Geometry: final body of the model. Coordinates: model frame, mm. Round coordinates to 2 decimals unless told otherwise and drop trailing zeros. Loops run counter-clockwise (first coordinate to the right, second up) from the corner with the lowest first, then second, coordinate; pieces in that order, holes last. Notation, with made-up numbers: M -2.5,-33.75 L 41.5,-33.75 A20 cw 41.5,-24.75 Z; hole C -9.5,-22 d3. An arc over 180 degrees is marked long. Write each question's results on one line, items separated by ' | '.
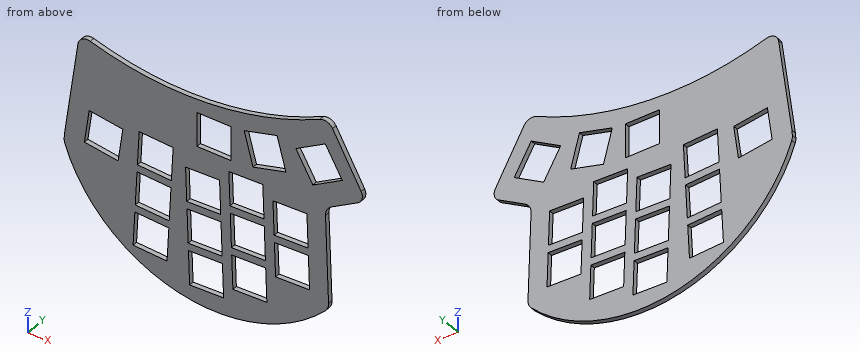
```python
from build123d import *

# Parameters (mm, degrees)
SKETCH1_W           = 14
SKETCH1_H           = 14
BOSS_EXTRUDE1_DEPTH = 2
FILLET1_R           = 5


with BuildPart() as part:
    # Sketch1 → Boss-Extrude1 (new body)
    with BuildSketch(Plane(origin=(0, 0, 0), x_dir=(1, 0, 0), z_dir=(0, 1, 0))):
        with BuildLine():
            Line((-10.586983819, 42.383324584), (-5.046266953, 2.959075179))
            ThreePointArc((-5.046266953, 2.959075179), (-3.174441029, 0.368828473), (0, 0))
            ThreePointArc((0, 0), (47.971062986, 5.333423777), (94.542026123, -7.347809821))
            ThreePointArc((94.542026123, -7.347809821), (97.488396157, -7.568143239), (99.777690602, -5.700317192))
            Line((99.777690602, -5.700317192), (111.550095971, 15.354261283))
            ThreePointArc((111.550095971, 15.354261283), (112.008410414, 17.939225635), (110.765402582, 20.251589006))
            Line((110.765402582, 20.251589006), (96.765402582, 28.334492774))
            Line((96.765402582, 28.334492774), (98.196951267, 69.32867968))
            ThreePointArc((98.196951267, 69.32867968), (36.880667069, 88.690951376), (-10.814532638, 45.566107052))
            Line((-10.814532638, 45.566107052), (-10.586983819, 42.383324584))
        make_face()
        Polygon((-0.449562029, 28.794432983), (13.414190971, 30.742856383), (11.465767571, 44.606609383), (-2.397985429, 42.658185983), align=None, mode=Mode.SUBTRACT)
        Polygon((20.152865671, 28.899486483), (34.133679071, 29.632189883), (33.400975671, 43.613003283), (19.420162271, 42.880299883), align=None, mode=Mode.SUBTRACT)
        Polygon((19.263154371, 45.876188583), (33.243967771, 46.608891983), (32.511264371, 60.589705383), (18.530450971, 59.857001983), align=None, mode=Mode.SUBTRACT)
        Polygon((18.373443071, 62.852890683), (32.354256471, 63.585594083), (31.621553071, 77.566407483), (17.640739671, 76.833704083), align=None, mode=Mode.SUBTRACT)
        Polygon((39.247799271, 35.544672383), (53.239270871, 35.056079383), (53.727863871, 49.047550983), (39.736392271, 49.536143983), align=None, mode=Mode.SUBTRACT)
        Polygon((39.841090671, 52.534316483), (53.832562271, 52.045723483), (54.321155271, 66.037195083), (40.329683671, 66.525788083), align=None, mode=Mode.SUBTRACT)
        Polygon((40.434382071, 69.523960583), (54.425853671, 69.035367583), (54.914446671, 83.026839183), (40.922975071, 83.515432183), align=None, mode=Mode.SUBTRACT)
        Polygon((57.062336771, 29.919527383), (71.053808371, 29.430934383), (71.542401371, 43.422405983), (57.550929771, 43.910998983), align=None, mode=Mode.SUBTRACT)
        Polygon((57.655628171, 46.909171483), (71.647099771, 46.420578483), (72.135692771, 60.412050083), (58.144221171, 60.900643083), align=None, mode=Mode.SUBTRACT)
        Polygon((58.248919571, 63.898815583), (72.240391171, 63.410222583), (72.728984171, 77.401694183), (58.737512571, 77.890287183), align=None, mode=Mode.SUBTRACT)
        Polygon((75.229359071, 34.388229583), (89.220830671, 33.899636583), (89.709423671, 47.891108183), (75.717952071, 48.379701183), align=None, mode=Mode.SUBTRACT)
        Polygon((75.822650471, 51.377873683), (89.814122071, 50.889280683), (90.302715071, 64.880752283), (76.311243471, 65.369345283), align=None, mode=Mode.SUBTRACT)
        with Locations((50.981291271, 18.033609783)):
            Rectangle(SKETCH1_W, SKETCH1_H, mode=Mode.SUBTRACT)
        Polygon((63.408077171, 10.383862283), (76.931038771, 6.760395683), (80.554505371, 20.283357283), (67.031543771, 23.906823883), align=None, mode=Mode.SUBTRACT)
        Polygon((96.794438284, 1.879855106), (103.794438261, 14.00421072), (91.670082648, 21.004210697), (84.670082671, 8.879855083), align=None, mode=Mode.SUBTRACT)
    extrude(amount=BOSS_EXTRUDE1_DEPTH)

    # Fillet1
    fillet1_edges = [part.edges().sort_by_distance(p)[0] for p in [
        (96.765402582, 1, -28.334492774),
        (-10.814532638, 1, -45.566107052),
        (98.196951267, 1, -69.32867968),
    ]]
    fillet(fillet1_edges, radius=FILLET1_R)


solid = part.part
```
1. Section B-B (z = -79.5). Output: boundary loops of the cut face in (x, y).
Answer key:
outline: M 15.07,0 L 40.78,0 L 40.78,2 L 15.07,2 Z; M 54.79,0 L 86.23,0 L 86.23,2 L 54.79,2 Z
2. Section C-C (y = 1.1). Count the separate pieces of the cut face and the enclosed holes in it, then the cut area to 3 significant figures.
Answer key:
separate pieces: 1 | enclosed holes: 15 | area: 5,750 mm²
3. Pin query (flat end, axial travel): P1, Ø1, axis at x = 53, y = 0.5, coming from the +Z side; P2, Ø1, axis at y = 1.5, z = -68, coming from the +X side. Return the tip coordinate at first contact, or that it passes through.
Answer key:
P1: stops at z = -4.78 | P2: stops at x = 98.13
4. Ray query, probe 1 along X at (y, z) = (0.85, -35); probe 2 along X at (y, z) = (0.4, -13); probe 3 along X at (y, z) = (1.4, -50.5). Return the intervals inside material, ascending.
Answer key:
probe 1: x = -9.55 to -1.32, 12.82 to 19.83, 33.85 to 57.24, 71.25 to 75.25, 89.26 to 97 | probe 2: x = -6.46 to 43.98, 57.98 to 64.11, 78.6 to 87.05, 103.21 to 110.23 | probe 3: x = -8.98 to 19.02, 33.04 to 57.78, 71.79 to 97.54
5. Section A-A (x = 49). Output: boundary loops of the cut face in (y, z), then the cut area to 3 significant figures.
Answer key:
outline: M 0,-90.15 L 2,-90.15 L 2,-83.23 L 0,-83.23 Z; M 0,-69.22 L 2,-69.22 L 2,-66.22 L 0,-66.22 Z; M 0,-52.21 L 2,-52.21 L 2,-49.21 L 0,-49.21 Z; M 0,-35.2 L 2,-35.2 L 2,-25.03 L 0,-25.03 Z; M 0,-11.03 L 2,-11.03 L 2,-5.25 L 0,-5.25 Z | area: 57.8 mm²
6. Section D-D (x = 27.5). Output: boundary loops of the cut face in (y, z).
Answer key:
outline: M 0,-85.89 L 2,-85.89 L 2,-77.35 L 0,-77.35 Z; M 0,-63.33 L 2,-63.33 L 2,-60.33 L 0,-60.33 Z; M 0,-46.31 L 2,-46.31 L 2,-43.3 L 0,-43.3 Z; M 0,-29.28 L 2,-29.28 L 2,-5.29 L 0,-5.29 Z
